```python
from build123d import *

# Parameters (mm, degrees)
F0_R          = 1
F1_DEPTH      = 1
F2_R          = 1.5
F3_SIZE       = 3
F4_R          = 1.5
F6_DEPTH      = 19.75
F6_DEPTH_BACK = 1
F9_R          = 1
F10_DEPTH     = 1.5
F11_W         = 20
F11_H         = 39.5
F11_R         = 1
F12_DEPTH     = 0.5


with BuildPart() as f1:
    # F0 (on Top) → F1 (new body)
    with BuildSketch(Plane.XY):
        with BuildLine():
            ThreePointArc((5.05, 0), (0, -5.05), (-5.05, 0))
            Line((-5.05, 0), (-5.05, 2.5))
            Line((-5.05, 2.5), (-9.5, 2.5))
            Line((-9.5, 2.5), (-9.5, 0))
            Line((-9.5, 0), (-9.5, -7))
            Line((-9.5, -7), (-5.853407529, -17.0189304721))
            Line((-5.853407529, -17.0189304721), (19.146592471, -23.7176602829))
            Line((19.146592471, -23.7176602829), (82.3319984622, -86.9030662741))
            Line((82.3319984622, -86.9030662741), (103.5452018978, -108.1162697097))
            Line((103.5452018978, -108.1162697097), (107.0807358037, -104.5807358037))
            Line((107.0807358037, -104.5807358037), (9.5, -7))
            Line((9.5, -7), (9.5, 0))
            Line((9.5, 0), (9.5, 2.5))
            Line((9.5, 2.5), (5.05, 2.5))
            Line((5.05, 2.5), (5.05, 0))
        make_face()
        with Locations((0, -7)):
            Circle(F0_R, mode=Mode.SUBTRACT)
        with Locations((-4.9497474683, -4.9497474683)):
            Circle(F0_R, mode=Mode.SUBTRACT)
        with Locations((-7, 0)):
            Circle(F0_R, mode=Mode.SUBTRACT)
        with Locations((4.9497474683, -4.9497474683)):
            Circle(F0_R, mode=Mode.SUBTRACT)
        with Locations((7, 0)):
            Circle(F0_R, mode=Mode.SUBTRACT)
        Polygon((89.4030662741, -122.2584053334), (103.5452018978, -108.1162697097), (82.3319984622, -86.9030662741), align=None)
    extrude(amount=F1_DEPTH)

    # F2
    f2_edges = [f1.edges().sort_by_distance(p)[0] for p in [
        (89.403066, -122.258405, 0.5),
        (82.331998, -86.903066, 0.5),
        (107.080736, -104.580736, 0.5),
        (19.146592, -23.71766, 0.5),
        (9.5, -7, 0.5),
        (9.5, 2.5, 0.5),
        (-5.05, 2.5, 0.5),
        (5.05, 2.5, 0.5),
        (-9.5, 2.5, 0.5),
        (-9.5, -7, 0.5),
    ]]
    fillet(f2_edges, radius=F2_R)

    # F3
    f3_edges = [f1.edges().sort_by_distance(p)[0] for p in [
        (-5.853408, -17.01893, 0.5),
    ]]
    chamfer(f3_edges, length=F3_SIZE)

    # F4
    f4_edges = [f1.edges().sort_by_distance(p)[0] for p in [
        (-6.879468, -14.199853, 0.5),
        (-2.95563, -17.795388, 0.5),
    ]]
    fillet(f4_edges, radius=F4_R)

    # F5 (on face) → F6 (join, two sides)
    with BuildSketch(Plane.XY.offset(1)) as f6_sk:
        Polygon((19.7530483272, -15.1317279836), (18.6923881554, -16.1923881554), (32.8345237792, -30.3345237792), (33.8951839509, -29.2738636074), align=None)
        Polygon((85.8675323681, -83.3675323681), (100.0096679919, -97.5096679919), (101.0703281637, -96.4490078201), (86.9281925399, -82.3068721964), align=None)
    extrude(amount=F6_DEPTH)
    extrude(f6_sk.sketch, amount=-F6_DEPTH_BACK)

    # F8: F1 across plane


with BuildPart() as f1_1:
    add(f1.part)
    add(f1.part.mirror(Plane(origin=(26.2937860532, -22.7331258814, 20.75), x_dir=(1, 0, 0), z_dir=(0, 0, 1))))

    # F9 (on face) → F10 (cut, through all)
    with BuildSketch(Plane(origin=(2.3106601718, 2.3106601718, 0), x_dir=(-0.7071067812, 0.7071067812, 0), z_dir=(0.7071067812, 0.7071067812, 0))):
        with Locations((-27.1672618896, 32.25)):
            Circle(F9_R)
        with Locations((-27.1672618896, 9.25)):
            Circle(F9_R)
        with Locations((-42.1672618896, 32.25)):
            Circle(F9_R)
        with Locations((-42.1672618896, 9.25)):
            Circle(F9_R)
        with Locations((-137.1672618896, 32.25)):
            Circle(F9_R)
        with Locations((-137.1672618896, 9.25)):
            Circle(F9_R)
        with Locations((-122.1672618896, 9.25)):
            Circle(F9_R)
        with Locations((-122.1672618896, 32.25)):
            Circle(F9_R)
    extrude(amount=-F10_DEPTH, mode=Mode.SUBTRACT)

    # F11 (on face) → F12 (cut)
    with BuildSketch(Plane(origin=(1.25, 1.25, 0), x_dir=(0.7071067812, -0.7071067812, 0), z_dir=(-0.7071067812, -0.7071067812, 0))):
        with Locations((34.6672618896, 20.75)):
            Rectangle(F11_W, F11_H)
        with Locations((27.1672618898, 9.25)):
            Circle(F11_R, mode=Mode.SUBTRACT)
        with Locations((42.1672618897, 9.25)):
            Circle(F11_R, mode=Mode.SUBTRACT)
        with Locations((27.1672618898, 32.25)):
            Circle(F11_R, mode=Mode.SUBTRACT)
        with Locations((42.1672618897, 32.25)):
            Circle(F11_R, mode=Mode.SUBTRACT)
        with Locations((129.6672618896, 20.75)):
            Rectangle(F11_W, F11_H)
        with Locations((122.1672618897, 9.25)):
            Circle(F11_R, mode=Mode.SUBTRACT)
        with Locations((137.1672618897, 9.25)):
            Circle(F11_R, mode=Mode.SUBTRACT)
        with Locations((122.1672618897, 32.25)):
            Circle(F11_R, mode=Mode.SUBTRACT)
        with Locations((137.1672618897, 32.25)):
            Circle(F11_R, mode=Mode.SUBTRACT)
    extrude(amount=-F12_DEPTH, mode=Mode.SUBTRACT)


solid = f1_1.part
```
CAD build for the part. Positions are in the model's coordinates, mm. A direction names the side the tool comes from. Round coordinates to 2 decimals unless told otherwise and drop trailing zeros. Loops run counter-clockwise (first coordinate to the right, second up) from the corner with the lowest first, then second, coordinate; pieces in that order, holes last. Notation, with made-up numbers: M 87.25,88 L 94.25,88 A20 cw 94.25,102 Z; hole C 14.25,3 d4. An arc over 180 degrees is marked long. Return JSON: item names as keys, results as strings. Group by question number.
(1) Saw through at B-B, the plane x = 76. List the corners of the cut face in (y, z), and give its area (3 significant figures).
(2) Mould opens along X. For faces 1 (the cylindrical face through (0.11, -5.05, 0.49)), 2 (the flat face through (7.929, -20.712, 41.007)), 3 (the flat face through (26.92, -22.3, 20.46)) say: +X half, -X half, draft (parallel to the pull), parting line (faces both ways), or undercut.
(3) Saw through at A-A, the plane z = 6. List the corners of the cut face in (x, y), and give its area (3 significant figures).
(4) Wall check: probe 1 along Z at (x, y) = (92.5, -114); probe 2 along Y at (x, z) = (31, 18.5); probe 3 along X at (y, z) = (-16.5, 23.5). Give the ranges that are in metal, low to high. Write a range as [from, to].
(5) Drop flat-ended pins along their axis: P1, Ø0.5, axis at y = -1.5, z = 41, coming from the +X side; P2, Ø1.5, axis at x = 23.5, z = 34.5, coming from the +Y side; P3, Ø2.5, axis at x = 7, y = 0, coming from the -Z side; P4, Ø10, axis at x = 25.5, z = 16, coming from the -Y side. Give the stop position or say it passes through.
(6) Tool access for faces 4 (the flat face through (53, -55, 1)), 5 (the flat face through (103.1, -100.6, 41)), 6 (the flat face through (57, -59, 0)): list every direction of +Z, -Z, +X, -X, +Y, -Y with a clear straight run to the whole face (end or side of a thin tool).
Answer list:
{
 "1": {"outline": "M -80.57,0 L -73.5,0 L -73.5,1 L -80.57,1 Z; M -80.57,40.5 L -73.5,40.5 L -73.5,41.5 L -80.57,41.5 Z", "area": "14.1 mm2"},
 "2": {"face 1": "undercut", "face 2": "-X half", "face 3": "+X half"},
 "3": {"outline": "M 19.05,-15.84 L 33.19,-29.98 L 33.9,-29.27 L 19.75,-15.13 Z; M 86.22,-83.01 L 100.36,-97.16 L 101.07,-96.45 L 86.93,-82.31 Z", "area": "40.0 mm2"},
 "4": {"probe 1": "[0, 1], [40.5, 41.5]", "probe 2": "[-27.79, -26.38]", "probe 3": "[19.71, 21.12]"},
 "5": {"P1": "x = 9.5", "P2": "y = -18.13", "P3": "z = 0", "P4": "y = -27.29"},
 "6": {"face 4": "-X, -Y", "face 5": "+Z, -Z, +X", "face 6": "-Z, +X, -X, +Y, -Y"}
}
